from build123d import *

# Parameters (mm, degrees)
BOSS_EXTRUDE1_DEPTH = 8
SKETCH2_R           = 4.75
CUT_EXTRUDE1_DEPTH  = 201.81338663
SKETCH3_R           = 2.159
CUT_EXTRUDE2_DEPTH  = 201.81338663
SKETCH4_R           = 3.175
CUT_EXTRUDE3_DEPTH  = 201.81338663
SKETCH5_R           = 2.159
CUT_EXTRUDE4_DEPTH  = 201.81338663


with BuildPart() as part:
    # Sketch1 → Boss-Extrude1 (new body)
    with BuildSketch(Plane(origin=(0, 0, 0), x_dir=(1, 0, 0), z_dir=(0, 1, 0))):
        with BuildLine():
            Line((-174.625, 12.7), (174.625, 12.7))
            ThreePointArc((174.625, 12.7), (200.025, 0), (174.625, -12.7))
            Line((174.625, -12.7), (-174.625, -12.7))
            ThreePointArc((-174.625, -12.7), (-200.025, 0), (-174.625, 12.7))
        make_face()
    extrude(amount=BOSS_EXTRUDE1_DEPTH)

    # Sketch2 → Cut-Extrude1 (cut, through all)
    with BuildSketch(Plane(origin=(0, 8, 0), x_dir=(1, 0, 0), z_dir=(0, 1, 0))):
        with Locations(Location((184.15, 0, 0), (0, 0, 270))):
            Circle(SKETCH2_R)
        with Locations(Location((-184.15, 0, 0), (0, 0, 90))):
            Circle(SKETCH2_R)
        with BuildLine():
            Line((173.691383345, 1.375), (175.608616655, 1.375))
            ThreePointArc((175.608616655, 1.375), (176.983616655, 0), (175.608616655, -1.375))
            Line((175.608616655, -1.375), (173.691383345, -1.375))
            ThreePointArc((173.691383345, -1.375), (172.316383345, 0), (173.691383345, 1.375))
        make_face()
        with BuildLine():
            Line((194.608616655, 1.375), (192.691383345, 1.375))
            ThreePointArc((192.691383345, 1.375), (191.316383345, 0), (192.691383345, -1.375))
            Line((192.691383345, -1.375), (194.608616655, -1.375))
            ThreePointArc((194.608616655, -1.375), (195.983616655, 0), (194.608616655, 1.375))
        make_face()
        with BuildLine():
            Line((185.525, 8.25), (185.525, 7.75))
            ThreePointArc((185.525, 7.75), (184.15, 6.375), (182.775, 7.75))
            Line((182.775, 7.75), (182.775, 8.25))
            ThreePointArc((182.775, 8.25), (184.15, 9.625), (185.525, 8.25))
        make_face()
        with BuildLine():
            Line((185.525, -8.25), (185.525, -7.75))
            ThreePointArc((185.525, -7.75), (184.15, -6.375), (182.775, -7.75))
            Line((182.775, -7.75), (182.775, -8.25))
            ThreePointArc((182.775, -8.25), (184.15, -9.625), (185.525, -8.25))
        make_face()
        with BuildLine():
            Line((-185.525, -8.25), (-185.525, -7.75))
            ThreePointArc((-185.525, -7.75), (-184.15, -6.375), (-182.775, -7.75))
            Line((-182.775, -7.75), (-182.775, -8.25))
            ThreePointArc((-182.775, -8.25), (-184.15, -9.625), (-185.525, -8.25))
        make_face()
        with BuildLine():
            Line((-185.525, 8.25), (-185.525, 7.75))
            ThreePointArc((-185.525, 7.75), (-184.15, 6.375), (-182.775, 7.75))
            Line((-182.775, 7.75), (-182.775, 8.25))
            ThreePointArc((-182.775, 8.25), (-184.15, 9.625), (-185.525, 8.25))
        make_face()
        with BuildLine():
            Line((-194.608616655, 1.375), (-192.691383345, 1.375))
            ThreePointArc((-192.691383345, 1.375), (-191.316383345, 0), (-192.691383345, -1.375))
            Line((-192.691383345, -1.375), (-194.608616655, -1.375))
            ThreePointArc((-194.608616655, -1.375), (-195.983616655, 0), (-194.608616655, 1.375))
        make_face()
        with BuildLine():
            Line((-173.691383345, 1.375), (-175.608616655, 1.375))
            ThreePointArc((-175.608616655, 1.375), (-176.983616655, 0), (-175.608616655, -1.375))
            Line((-175.608616655, -1.375), (-173.691383345, -1.375))
            ThreePointArc((-173.691383345, -1.375), (-172.316383345, 0), (-173.691383345, 1.375))
        make_face()
    extrude(amount=-CUT_EXTRUDE1_DEPTH, mode=Mode.SUBTRACT)

    # Sketch3 → Cut-Extrude2 (cut, through all)
    with BuildSketch(Plane(origin=(0, 8, 0), x_dir=(1, 0, 0), z_dir=(0, 1, 0))):
        with Locations(Location((0, 0, 0), (0, 0, 270))):
            Circle(SKETCH3_R)
        with Locations(Location((38.1, 0, 0), (0, 0, 270))):
            Circle(SKETCH3_R)
        with Locations(Location((-38.1, 0, 0), (0, 0, 270))):
            Circle(SKETCH3_R)
    extrude(amount=-CUT_EXTRUDE2_DEPTH, mode=Mode.SUBTRACT)

    # Sketch4 → Cut-Extrude3 (cut, through all)
    with BuildSketch(Plane(origin=(0, 8, 0), x_dir=(1, 0, 0), z_dir=(0, 1, 0))):
        with Locations(Location((-19.05, 0, 0), (0, 0, 270))):
            Circle(SKETCH4_R)
        with Locations(Location((19.05, 0, 0), (0, 0, 270))):
            Circle(SKETCH4_R)
    extrude(amount=-CUT_EXTRUDE3_DEPTH, mode=Mode.SUBTRACT)

    # Sketch5 → Cut-Extrude4 (cut, through all)
    with BuildSketch(Plane(origin=(0, 8, 0), x_dir=(1, 0, 0), z_dir=(0, 1, 0))):
        with Locations(Location((54.61, 0, 0), (0, 0, 270))):
            Circle(SKETCH5_R)
        with Locations(Location((-54.61, 0, 0), (0, 0, 90))):
            Circle(SKETCH5_R)
    extrude(amount=-CUT_EXTRUDE4_DEPTH, mode=Mode.SUBTRACT)


solid = part.part
The model under review builds one solid part; all positions refer to its coordinate system, in mm. A direction names the side the tool comes from. Give positions to 0.01 mm unless a question says otherwise; leave off trailing zeros. Answer as a JSON object with one key per item and string values. Group by question number.
Q1. Take a section at A-A (y = 5.25). State how many separate pieces and enclosed holes the cut face has, plus the area to 3 significant figures.
Q2. Draft analysis for pull direction X (two halves, no side actions). For faces 1 (the cylindrical face through (15.95, 4.06, -0.69)), 2 (the flat face through (3, 0, 0)), state which applies: pulls with the +X half, pulls with the -X half, needs draft (parallel to the pull), parting line crosses it, or undercut.
Q3. Wall thickness on line 1 along Z through (x, y) = (-54.61, 5.5); line 2 along X through (y, z) = (4.25, -6.5); line 3 along Z through (x, y) = (-184.15, 2) (3 decimals): over which ranges is each line inside the solid? List them lowest first.
Q4. Insertion check: pin 1 (1 mm diameter, centred on x = -193, y = 2.5, fed in from +Z); pin 2 (0.6 mm diameter, centred on y = 5, z = 8, fed in from -X); pin 3 (4 mm diameter, centred on x = 32.5, y = 2.5, fed in from -Z); pin 4 (8.5 mm diameter, centred on x = 184.15, z = 0, fed in from -Y). Each pin has a flat end and moves straight along its axis. Give the tip position at first contact, or say it passes through.
Q5. Tool access review of faces 3 (the flat face through (2, 4, 12.7)), 4 (the cylindrical face through (200.017, 3.944, -0.492)), 5 (the flat face through (-2, 4, -12.7)): name each direction out of +Z, -Z, +X, -X, +Y, -Y from which nothing blocks a thin tool from reaching the whole face with its end or side.
Answer below:
{
 "1": {"separate pieces": "1", "enclosed holes": "17", "area": "9,880 mm2"},
 "2": {"face 1": "undercut", "face 2": "needs draft"},
 "3": {"line 1": "z = -12.7 to -2.16, 2.16 to 12.7", "line 2": "x = -198.63 to -184.72, -183.58 to 183.58, 184.72 to 198.63", "line 3": "z = -15.875 to -9.625, -6.375 to -4.75, 4.75 to 6.375, 9.625 to 15.875"},
 "4": {"pin 1": "stops at z = 13.5", "pin 2": "stops at x = -198.03", "pin 3": "stops at z = -12.7", "pin 4": "passes through"},
 "5": {"face 3": "+Z, +Y, -Y", "face 4": "+Y, -Y", "face 5": "-Z, +Y, -Y"}
}
